Verification items for the finished model (mm, model axes). Face numbers are marked on the shaded views. A direction names the side the tool comes from. Round coordinates to 2 decimals unless told otherwise and drop trailing zeros. Loops run counter-clockwise (first coordinate to the right, second up) from the corner with the lowest first, then second, coordinate; pieces in that order, holes last. Notation, with made-up numbers: M 23.5,-0.5 L 65.5,-0.5 A17 ccw 65.5,26.5 Z; hole C -28,60 d9. An arc over 180 degrees is marked long. Answer as CSV lines item,"result".
Autodesk Inventor part; units mm, degrees
ref_plane "Work Plane1" through (-11, -21.5, 0) normal (-1, 0, 0) x (0, 0, 1)
ref_plane "YZ Plane" through (0, 0, 0) normal (1, 0, 0) x (0, 1, 0)
ref_plane "XZ Plane" through (0, 0, 0) normal (0, 1, 0) x (-1, 0, 0)
sketch "Sketch1" plane through (0, 0, 0) normal (0, 0, 1) x (1, 0, 0)
  line L0 (-10, -21.5) -> (10, -21.5)
  line L1 (10, -21.5) -> (10, 21.5)
  line L2 (10, 21.5) -> (-10, 21.5)
  line L3 (-10, 21.5) -> (-10, -21.5)
  line L4 (-10, -21.5) -> (10, 21.5) construction
  line L5 (10, -21.5) -> (-10, 21.5) construction
  point P0 (0, 0)
  dimension "d0" = 20
  dimension "d1" = 43
extrude "Extrusion1" add sketch "Sketch1" along normal blind 3.5
sketch "Sketch2" plane through (0, 0, 3.5) normal (0, 0, 1) x (1, 0, 0)
  line L0 (-7.5, -8) -> (7.5, -8)
  line L1 (7.5, -8) -> (7.5, 8)
  line L2 (7.5, 8) -> (-7.5, 8)
  line L3 (-7.5, 8) -> (-7.5, -8)
  line L4 (-7.5, -8) -> (7.5, 8) construction
  line L5 (7.5, -8) -> (-7.5, 8) construction
  point P0 (0, 0)
  dimension "d4" = 15
  dimension "d5" = 16
hole "Hole1" at (-7.5, 8, 3.5) at (7.5, 8, 3.5) at (7.5, -8, 3.5) at (-7.5, -8, 3.5) direction (0, 0, -1) diameter 3 end through all
sketch "Sketch3" plane through (10, -21.5, 0) normal (1, 0, 0) x (0, 0, -1)
  circle A0 centre (3.5, 30.5) radius 11.9062
  line L0 (0, 0) -> (0, 43)
  circle A1 centre (3.5, 30.5) radius 12.5
  line L1 (0, 43) -> (3.5, 43)
  line L2 (14.2623, 24.142) -> (0, 0)
  line L3 (-3.5, 43) -> (-3.5, 0)
  line L4 (-3.5, 43) -> (-7.1577, 37.0317)
  line L5 (-3.5, 0) -> (-8.786, 28.1968)
  line L6 (0, 0) -> (-3.5, 0)
  line L7 (0, 43) -> (-3.5, 43)
  line L8 (16, 30.5) -> (16, 43)
  line L9 (16, 43) -> (-9, 43)
  line L10 (-9, 43) -> (-9, 30.5)
  line L11 (9, 43) -> (12.7158, 38.945)
  point P0 (0, 21.5)
  point P1 (0, 21.5)
  point P2 (3.5, 43)
  dimension "d14" = 25
  dimension "d13" = 23.8125
  dimension "d15" = 3.5
  dimension "d26" = 9
extrude "Extrusion2" add sketch "Sketch3" along normal blind 3.5
sketch "Sketch4" plane through (13.5, -21.5, 0) normal (1, 0, 0) x (0, 0, -1)
  circle A0 centre (3.5, 30.5) radius 11.9062
  point P0 (0, 21.5)
extrude "Extrusion3" add sketch "Sketch4" along normal blind 0.5
sketch "Sketch5" plane through (10, -21.5, 0) normal (-1, 0, 0) x (0, 0, 1)
  line L0 (3.5, 0) -> (3.5, 43)
  line L1 (8.786, 28.1968) -> (3.5, 0)
  arc A0 (-16, 30.5) -> (-14.2623, 24.142) centre (-3.5, 30.5) ccw
  arc A1 (8.786, 28.1968) -> (9, 30.5) centre (-3.5, 30.5) ccw
  line L2 (0, 0) -> (0, 43)
  line L3 (0, 0) -> (-14.2623, 24.142)
  line L4 (-16, 43) -> (0, 43)
  line L5 (-16, 30.5) -> (-16, 43)
  line L6 (9, 43) -> (9, 30.5)
  line L7 (3.5, 43) -> (9, 43)
  point P0 (0, 21.5)
extrude "Extrusion4" add sketch "Sketch5" along normal blind 0.25
sketch "Sketch6" plane through (10, -21.5, 0) normal (-1, 0, 0) x (0, 0, 1)
  line L0 (-14.2623, 24.142) -> (0, 0)
  line L1 (0, 43) -> (0, 0)
  line L2 (0, 43) -> (-16, 43)
  line L3 (-16, 43) -> (-16, 30.5)
  arc A0 (-16, 30.5) -> (-14.2623, 24.142) centre (-3.5, 30.5) ccw
  line L4 (-8, 13.5418) -> (-8, 43)
  dimension "d67" = 8
extrude "Extrusion5" add sketch "Sketch6" along normal blind 5 contours A0 L3 L2 L4 L0
sketch "Sketch7" plane through (14, 9, -3.5) normal (1, 0, 0) x (0, 0, -1)
  circle A0 centre (0, 0) radius 11.9062
  circle A1 centre (0, 0) radius 6.1
  circle A2 centre (-2, 3.4641) radius 1.5
  circle A3 centre (4, 0) radius 1.5
  circle A4 centre (-2, -3.4641) radius 1.5
  line L0 (-2, 3.4641) -> (0, 0) construction
  line L1 (0, 0) -> (4, 0) construction
  line L2 (-2, -3.4641) -> (0, 0) construction
  circle A5 centre (0, 0) radius 2
  point P0 (-3.5, -9)
  dimension "d27" = 12.2
  dimension "d28" = 3
  dimension "d29" = 120
  dimension "d30" = 120
  dimension "d31" = 4
  dimension "d32" = 4
sketch "Sketch10" plane through (14, 9, -3.5) normal (1, 0, 0) x (0, 0, -1)
  circle A0 centre (0, 0) radius 11.9062
  circle A1 centre (0, 0) radius 6.1
  point P0 (-3.5, -9)
  dimension "d44" = 12.2
extrude "Extrusion7" add sketch "Sketch10" along normal blind 5.28 contours A1
sketch "Sketch11" plane through (19.28, 9, -3.5) normal (1, 0, 0) x (0, 0, -1)
  circle A0 centre (0, 0) radius 6.1
  circle A1 centre (0, 0) radius 4
  point P0 (-3.5, -9)
  dimension "d47" = 8
extrude "Extrusion8" add sketch "Sketch11" along normal blind 5 contours A1
sketch "Sketch12" plane through (24.28, 9, -3.5) normal (1, 0, 0) x (0, 0, -1)
  circle A0 centre (0, 0) radius 4
  point P0 (-3.5, -9)
hole "Hole3" at (24.28, 9, -3.5) direction (-1, 0, 0) diameter 4 end through all
sketch "Sketch13" plane through (10, -21.5, 0) normal (-1, 0, 0) x (0, 0, 1)
  circle A0 centre (-3.5, 30.5) radius 2
  line L0 (-8, 43) -> (-8, 13.5418)
  line L1 (-8, 13.5418) -> (0, 0)
  line L2 (0, 43) -> (0, 0)
  line L3 (0, 43) -> (-8, 43)
  line L4 (-7, 32.5207) -> (-3.5, 34.5415)
  line L5 (-3.5, 34.5415) -> (0, 32.5207)
  line L6 (0, 32.5207) -> (0, 28.4793)
  line L7 (0, 28.4793) -> (-3.5, 26.4585)
  line L8 (-3.5, 26.4585) -> (-7, 28.4793)
  line L9 (-7, 28.4793) -> (-7, 32.5207)
  point P0 (-7, 30.5)
  point P1 (0, 28.4793)
  point P2 (0, 32.5207)
  dimension "d68" = 7
extrude "Extrusion9" cut sketch "Sketch13" against normal blind 3.7 contours L2 L7 L8 L9 L4 L5
sketch "Sketch15" plane through (19.28, 9, -3.5) normal (1, 0, 0) x (0, 0, -1)
  circle A0 centre (0, 0) radius 4
  circle A1 centre (0, 0) radius 6.1
  line L0 (3.75, 4.8112) -> (-3.75, 4.8112)
  point P0 (-3.5, -9)
  dimension "d62" = 7.5
extrude "Extrusion11" cut sketch "Sketch15" against normal up to surface (5.28 mm away) contours L0 A1 picked at (-0.8686, 5.0459)
sketch "Sketch17" plane through (9.75, -21.5, 0) normal (-1, 0, 0) x (0, 0, 1)
  line L0 (-7, 28.4793) -> (-7, 32.5207)
  line L1 (-3.5, 26.4585) -> (-7, 28.4793)
  line L2 (0, 28.4793) -> (-3.5, 26.4585)
  line L3 (0, 32.5207) -> (0, 28.4793)
  line L4 (-3.5, 34.5415) -> (0, 32.5207)
  line L5 (-7, 32.5207) -> (-3.5, 34.5415)
  circle A0 centre (-3.5, 30.5) radius 2
  point P0 (0, 21.5)
extrude "Extrusion13" cut sketch "Sketch17" against normal blind 3.7 contours L0 L5 L4 L3 L2 L1 | A0
fillet "Fillet2" radius 1 1 edges at (7.375, -7.9582, -8)
sketch "Sketch18" plane through (9.75, -21.5, 0) normal (-1, 0, 0) x (0, 0, 1)
  line L0 (0, 28.4793) -> (-3.5, 26.4585)
  line L1 (-3.5, 26.4585) -> (-7, 28.4793)
  line L2 (-7, 28.4793) -> (-7, 32.5207)
  line L3 (-7, 32.5207) -> (-3.5, 34.5415)
  line L4 (-3.5, 34.5415) -> (0, 32.5207)
  line L5 (0, 43) -> (0, 32.5207)
  line L6 (0, 43) -> (-8, 43)
  line L7 (-8, 43) -> (-8, 17.2005)
  arc A0 (-9.861, 16.6919) -> (-8, 17.2005) centre (-9, 17.2005) ccw
  line L8 (-9.861, 16.6919) -> (0, 0)
  line L9 (0, 28.4793) -> (0, 0)
  point P0 (0, 21.5)
extrude "Extrusion14" cut sketch "Sketch18" against normal blind 0.25
ref_plane "Work Plane1" through (-11, -21.5, 0) normal (-1, 0, 0) x (0, 0, 1)
mirror "Mirror1" about plane through (-11, -21.5, 0) normal (-1, 0, 0) of "Extrusion1", "Hole1", "Extrusion2", "Extrusion3", "Extrusion4", "Extrusion5", "Extrusion7", "Extrusion8", "Hole3", "Extrusion9", "Extrusion11", "Extrusion13", "Fillet2", "Extrusion14"
sketch "Sketch19" plane through (-11, -21.5, 0) normal (-1, 0, 0) x (0, 0, 1)
  line L0 (-26.4701, -15.0074) -> (17.4098, -15.0074)
  line L1 (17.4098, -15.0074) -> (17.4098, 56.4974)
  line L2 (17.4098, 56.4974) -> (-26.4701, 56.4974)
  line L3 (-26.4701, 56.4974) -> (-26.4701, -15.0074)
  point P0 (0, 21.5)
extrude "Extrusion15" cut sketch "Sketch19" against normal through all
equation "\"d30\" = d29"
properties part number "CarriagePivotMountMirror" material "ABS Plastic"
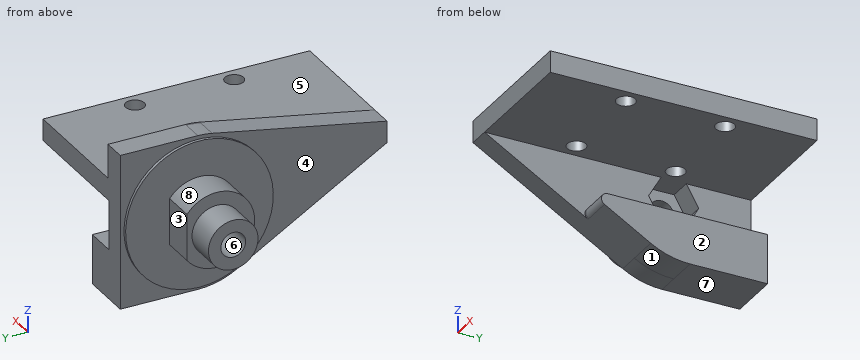
1) Section check B-B (x = -29.5). Record the cut outline in (y, z).
Here are the results:
outline,"M -21.5,0 L -9.5,0 L -9.5,3.5 L -21.5,3.5 Z; M -6.5,0 L 6.5,0 L 6.5,3.5 L -6.5,3.5 Z; M -4.81,-9.86 L 2.64,-14.26 A12.5 ccw 9,-16 L 21.5,-16 L 21.5,-8 L -4.3,-8 A1 ccw Z; M 9.5,0 L 21.5,0 L 21.5,3.5 L 9.5,3.5 Z"
2) Material ranges on probe 1 along Y at (x, z) = (-14.5, 2.8); probe 2 along X at (y, z) = (-8, 0.85); probe 3 along X at (y, z) = (8, 2.1), recorded low to high.
Here are the results:
probe 1,"y = -21.5 to -9.5, -6.5 to 6.5, 9.5 to 21.5"
probe 2,"x = -35.5 to -31, -28 to -16, -13 to -12"
probe 3,"x = -41.28 to -31, -28 to -16, -13 to -12"
3) Section check A-A (x = -14.5). Record the cut outline in (y, z), plus the area to 4 significant figures.
Here are the results:
outline,"M -21.5,0 L -9.5,0 L -9.5,3.5 L -21.5,3.5 Z; M -6.5,0 L 6.5,0 L 6.5,3.5 L -6.5,3.5 Z; M 9.5,0 L 21.5,0 L 21.5,3.5 L 9.5,3.5 Z"
area,"129.5 mm^2"
4) Section check C-C (z = -3). Record the cut outline in (x, y), plus the area to 3 significant figures.
Here are the results:
outline,"M -46.28,5.03 L -41.28,5.03 L -41.28,2.92 L -36,2.92 L -36,-2.9 L -35.5,-2.9 L -35.5,-16.42 L -32,-16.42 L -32,5.25 L -35.7,5.25 L -35.7,7.06 L -46.28,7.06 Z; M -46.28,10.94 L -35.7,10.94 L -35.7,12.75 L -32,12.75 L -32,21.5 L -35.5,21.5 L -35.5,20.9 L -36,20.9 L -36,13.81 L -41.28,13.81 L -41.28,12.97 L -46.28,12.97 Z"
area,"173 mm^2"
5) Draft check along Z on the marked faces 6, 7 and 8. Enter one of: +Z half, -Z half, draft (parallel to the pull), parting line (faces both ways), or undercut.
Here are the results:
face 6,"undercut"
face 7,"-Z half"
face 8,"parting line"
6) Set-up check for the marked faces 1, 2, 3, 4 and 5: record each of +Z, -Z, +X, -X, +Y, -Y from which the full face is reachable in a straight line by a thin tool's end or side.
Here are the results:
face 1,"-Z, +X, -X, -Y"
face 2,"-Z, +X, +Y, -Y"
face 3,"+Z, -Z, -X, +Y"
face 4,"-X"
face 5,"+Z, +X, +Y, -Y"
7) Section check D-D (y = -8). Record the cut outline in (x, z).
Here are the results:
outline,"M -35.5,-7.98 L -32,-7.98 L -32,0 L -31,0 L -31,3.5 L -31.75,3.5 L -31.75,6.03 L -35.5,6.03 Z; M -28,0 L -16,0 L -16,3.5 L -28,3.5 Z; M -13,0 L -12,0 L -12,3.5 L -13,3.5 Z"
8) Go/stop test with flat-tipped pins: pin 1 (6 mm diameter, centred on x = -39.5, z = -2.5, fed in from +Y); pin 2 (3.5 mm diameter, centred on x = -14.5, y = -8, fed in from -Z); pin 3 (1.5 mm diameter, centred on x = -29, y = 8.5, fed in from +Z); pin 4 (2.5 mm diameter, centred on x = -14.5, y = 8, fed in from -Z). Record where each tip stops, or that it passes through.
Here are the results:
pin 1,"stops at y = 13.81"
pin 2,"stops at z = 0"
pin 3,"stops at z = -8"
pin 4,"passes through"
